Here's how the part is built. I have some questions about the finished solid (model axes, mm). A direction names the side the tool comes from. Coordinates: 2 decimals unless noted, no trailing zeros. Loops run counter-clockwise (first coordinate to the right, second up) from the corner with the lowest first, then second, coordinate; pieces in that order, holes last. Notation, with made-up numbers: (39.5, 8.25) -> (83.5, 8.25) arc R24 cw to (83.5, 47.25) -> close; hole circle Ø5 at (85.25, 58). An arc over 180 degrees is marked (long way). Answer as a JSON object with one key per item and string values. Group by question number.
1) I want a section at A-A (y = 1.5). Count the separate pieces of the cut face and the enclosed holes in it, then the cut area to 3 significant figures.
2) I want a section at D-D (x = -37). Write out the boundary of the cut face in (y, z), then the cut area to 3 significant figures.
3) I need wall thicknesses on probe 1 along Y at (x, z) = (-9, -22); probe 2 along Y at (x, z) = (-24, 37); probe 3 along X at (y, z) = (1.25, 21.5). Which ranges of each line are inside material? Lowest first, please. Write a range as [from, to].
4) I want a section at B-B (z = -11). Write out the boundary of the cut face in (x, y).
5) Which directions (+Z, -Z, +X, -X, +Y, -Y) give clear straight access to the entire face, cutting with the end or side of a thin tool? Please do faces 1 (the flat face through (35, 3.81, -3)), 2 (the cylindrical face through (0.052, 2.576, 29.866)).
6) I want a section at C-C (x = 28). Write out the boundary of the cut face in (y, z).
7) I'm going to push flat-ended pins straight in: pin 1 (20.5 mm diameter, centred on x = 16.5, z = -6, fed in from +Y); pin 2 (3 mm diameter, centred on y = 4.5, z = -5, fed in from +X); pin 3 (1.4 mm diameter, centred on x = 0, z = 0, fed in from +Y); pin 4 (0.6 mm diameter, centred on x = -2, y = 8, fed in from -Z). Where does each tip first touch, or does it pass through?
8) If we mould it in two halves opening along Z, with no side actions, what happens to faces 3 (the cylindrical face through (-0.359, 2.576, -9.566)), 4 (the cylindrical face through (45.87, 1.88, 10.19)), 5 (the cylindrical face through (9.566, 2.576, -0.359)), 6 (the flat face through (0, 5.08, 7))? For each: +Z half, -Z half, draft (parallel to the pull), parting line (faces both ways), or undercut.
```python
from build123d import *

# Parameters (mm, degrees)
SKETCH1_R         = 46.99
EXTRUDE1_DEPTH    = 3.81
SKETCH2_R         = 34.29
EXTRUDE2_DEPTH    = 1.27
SKETCH3_R         = 4.445
EXTRUDE3_DEPTH    = 4.318
SKETCH4_R         = 1.1811
EXTRUDE4_DEPTH    = 68.115144371
SKETCH5_R         = 1.1938
SKETCH5_R_2       = 1.5875
EXTRUDE5_DEPTH    = 67.647780158
CIRPATTERN1_COUNT = 4
SKETCH6_R         = 2.8321
EXTRUDE6_DEPTH    = 4.318
EXTRUDE7_DEPTH    = 4.318
CIRPATTERN2_COUNT = 24


with BuildPart() as part:
    # Sketch1 → Extrude1 (new body)
    with BuildSketch(Plane(origin=(0, 0, 0), x_dir=(1, 0, 0), z_dir=(0, 1, 0))):
        with Locations(Location((0, 0, 0), (0, 0, 90))):
            Circle(SKETCH1_R)
    extrude(amount=EXTRUDE1_DEPTH)

    # Sketch2 → Extrude2 (add)
    with BuildSketch(Plane(origin=(0, 3.81, 0), x_dir=(1, 0, 0), z_dir=(0, 1, 0))):
        with Locations(Location((0, 0, 0), (0, 0, 270))):
            Circle(SKETCH2_R)
    extrude(amount=EXTRUDE2_DEPTH)

    # Sketch3 → Extrude3 (add)
    with BuildSketch(Plane(origin=(0, 5.08, 0), x_dir=(1, 0, 0), z_dir=(0, 1, 0))):
        with Locations(Location((0, 0, 0), (0, 0, 270))):
            Circle(SKETCH3_R)
    extrude(amount=EXTRUDE3_DEPTH)

    # Sketch4 → Extrude4 (cut, through all)
    with BuildSketch(Plane(origin=(0, 9.398, 0), x_dir=(1, 0, 0), z_dir=(0, 1, 0))):
        with Locations(Location((0, 0, 0), (0, 0, 270))):
            Circle(SKETCH4_R)
    extrude(amount=-EXTRUDE4_DEPTH, mode=Mode.SUBTRACT)

    # Sketch5 → Extrude5 (cut, through all)
    with BuildSketch(Plane(origin=(0, 5.08, 0), x_dir=(1, 0, 0), z_dir=(0, 1, 0))):
        with Locations(Location((0, -8.42772, 0), (0, 0, 270))):
            Circle(SKETCH5_R)
        with Locations(Location((0, -16.59382, 0), (0, 0, 270))):
            Circle(SKETCH5_R_2)
        with Locations(Location((0, -31.05912, 0), (0, 0, 270))):
            Circle(SKETCH5_R)
    extrude5 = extrude(amount=-EXTRUDE5_DEPTH, mode=Mode.SUBTRACT)

    # CirPattern1: Extrude5 ×4 about axis
    cirpattern1_axis = Axis((0, 0, 0), (0, 1, 0))
    for i in range(1, CIRPATTERN1_COUNT):
        add(extrude5.rotate(cirpattern1_axis, i * 360 / CIRPATTERN1_COUNT), mode=Mode.SUBTRACT)

    # Sketch6 → Extrude6 (cut)
    with BuildSketch(Plane(origin=(0, 9.398, 0), x_dir=(1, 0, 0), z_dir=(0, 1, 0))):
        with Locations(Location((0, 0, 0), (0, 0, 270))):
            Circle(SKETCH6_R)
    extrude(amount=-EXTRUDE6_DEPTH, mode=Mode.SUBTRACT)

    # Sketch7 → Extrude7 (add)
    with BuildSketch(Plane(origin=(0, 9.398, 0), x_dir=(1, 0, 0), z_dir=(0, 1, 0))):
        Polygon((0, 2.4384), (0.369663229, 2.807870992), (0.369663229, 3.102932626), (-0.369663229, 3.102932626), (-0.369663229, 2.807870992), align=None)
    extrude7 = extrude(amount=-EXTRUDE7_DEPTH)

    # CirPattern2: Extrude7 ×24 about axis
    cirpattern2_axis = Axis((0, 0, 0), (0, 1, 0))
    for i in range(1, CIRPATTERN2_COUNT):
        add(extrude7.rotate(cirpattern2_axis, i * 360 / CIRPATTERN2_COUNT))


solid = part.part
```
Determined:
{
 "1": {"separate pieces": "1", "enclosed holes": "13", "area": "6,860 mm^2"},
 "2": {"outline": "(0, -28.97) -> (3.81, -28.97) -> (3.81, 28.97) -> (0, 28.97) -> close", "area": "221 mm^2"},
 "3": {"probe 1": "[0, 5.08]", "probe 2": "[0, 3.81]", "probe 3": "[-41.78, 41.78]"},
 "4": {"outline": "(-45.68, 0) -> (45.68, 0) -> (45.68, 3.81) -> (32.48, 3.81) -> (32.48, 5.08) -> (-32.48, 5.08) -> (-32.48, 3.81) -> (-45.68, 3.81) -> close"},
 "5": {"face 1": "+Y", "face 2": "+Y, -Y"},
 "6": {"outline": "(0, -37.74) -> (3.81, -37.74) -> (3.81, -19.79) -> (5.08, -19.79) -> (5.08, 19.79) -> (3.81, 19.79) -> (3.81, 37.74) -> (0, 37.74) -> close"},
 "7": {"pin 1": "y = 5.08", "pin 2": "x = 46.85", "pin 3": "through", "pin 4": "z = -4.11"},
 "8": {"face 3": "undercut", "face 4": "parting line", "face 5": "undercut", "face 6": "draft"}
}
